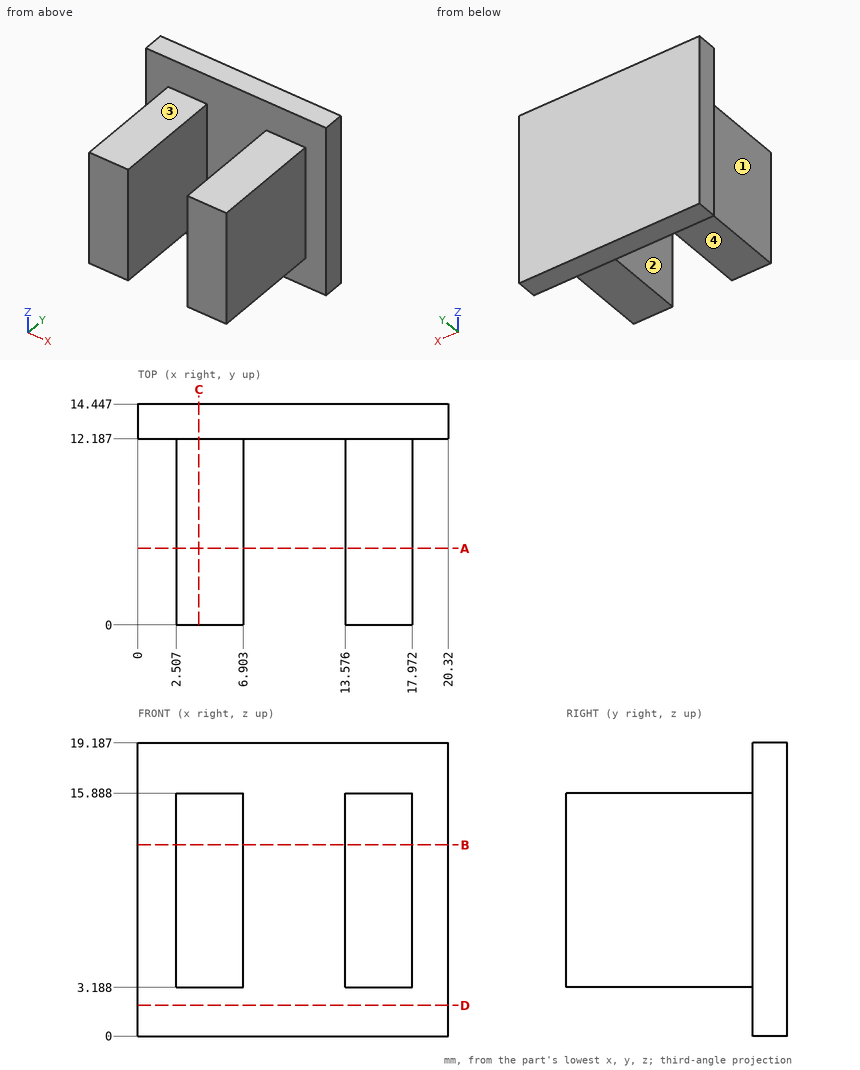
For this review, use the dimensioned drawing (mm, ordinates from the lowest corner) and the shaded views. A direction names the side the tool comes from. Give positions to 0.01 mm unless a question says otherwise; leave off trailing zeros. Write each loop counter-clockwise with the first axis right and the second up, starting at its lowest first coordinate (ties: lowest second). Pieces come first, ordered by that corner, then holes. Notation, with made-up numbers: M -15.75,43.5 L 10.25,43.5 A10 cw 10.25,54.5 Z; hole C 17.5,-23.5 d6. An arc over 180 degrees is marked long. Answer as a JSON object with one key per item and string values. Group by question number.
1) For line 1 along X through (y, z) = (4.25, 13.5); line 2 along Y through (x, z) = (13.5, 1.5); line 3 along Z through (x, y) = (4.5, 3.75), list the stretches that pass through material, from the lowest coordinate up.
2) We need section C-C (x = 4). Give the boundary of the cut face in (y, z), and give its area (3 significant figures).
3) We need section B-B (z = 12.5). Give the boundary of the cut face in (x, y), and give its area (3 significant figures).
4) We need section A-A (y = 5). Give the boundary of the cut face in (x, z), and give its area (3 significant figures).
5) We need section D-D (z = 2). Give the boundary of the cut face in (x, y).
6) Clearance check with flat-ended pins moving along their axes: pin 1 Ø3.5 at (y, z) = (4.5, 12) entering from +X; pin 2 Ø3 at (x, y) = (17.5, 9) entering from +Z; pin 3 Ø2 at (y, z) = (8, 3.5) entering from -X; pin 4 Ø4 at (x, z) = (7.5, 7.5) entering from -Y. State where each tip first meets the part, or that it passes through.
7) Tool access review of the marked faces 1, 2, 3 and 4: name each direction out of +Z, -Z, +X, -X, +Y, -Y from which nothing blocks a thin tool from reaching the whole face with its end or side.
Answer key:
{
 "1": {"line 1": "x = 2.51 to 6.9, 13.58 to 17.97", "line 2": "y = 12.19 to 14.45", "line 3": "z = 3.19 to 15.89"},
 "2": {"outline": "M 0,3.19 L 12.19,3.19 L 12.19,0 L 14.45,0 L 14.45,19.19 L 12.19,19.19 L 12.19,15.89 L 0,15.89 Z", "area": "198 mm²"},
 "3": {"outline": "M 0,12.19 L 2.51,12.19 L 2.51,0 L 6.9,0 L 6.9,12.19 L 13.58,12.19 L 13.58,0 L 17.97,0 L 17.97,12.19 L 20.32,12.19 L 20.32,14.45 L 0,14.45 Z", "area": "153 mm²"},
 "4": {"outline": "M 2.51,3.19 L 6.9,3.19 L 6.9,15.89 L 2.51,15.89 Z; M 13.58,3.19 L 17.97,3.19 L 17.97,15.89 L 13.58,15.89 Z", "area": "112 mm²"},
 "5": {"outline": "M 0,12.19 L 20.32,12.19 L 20.32,14.45 L 0,14.45 Z"},
 "6": {"pin 1": "stops at x = 17.97", "pin 2": "stops at z = 15.89", "pin 3": "stops at x = 2.51", "pin 4": "stops at y = 0"},
 "7": {"face 1": "+Z, -Z, -X, -Y", "face 2": "+Z, -Z, -Y", "face 3": "+Z, +X, -X, -Y", "face 4": "-Z, +X, -X, -Y"}
}
